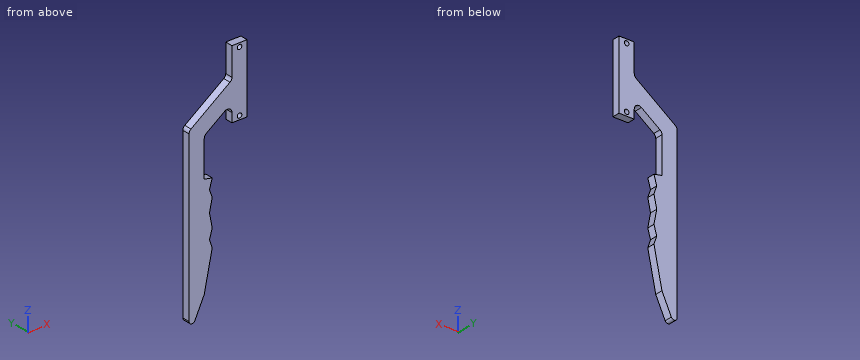
from build123d import *

# Parameters (mm, degrees)
SKETCH1_W           = 10
SKETCH1_H           = 45
BOSS_EXTRUDE1_DEPTH = 5
SKETCH2_R           = 1.5
CUT_EXTRUDE1_DEPTH  = 8
BOSS_EXTRUDE3_DEPTH = 5
BOSS_EXTRUDE4_DEPTH = 5
FILLET1_R           = 2
FILLET2_R           = 3
FILLET3_R           = 3


with BuildPart() as part:
    # Sketch1 → Boss-Extrude1 (new body)
    with BuildSketch(Plane(origin=(0, 0, 0), x_dir=(1, 0, 0), z_dir=(0, 1, 0))):
        Rectangle(SKETCH1_W, SKETCH1_H)
    extrude(amount=BOSS_EXTRUDE1_DEPTH)

    # Sketch2 → Cut-Extrude1 (cut)
    with BuildSketch(Plane(origin=(0, 5, 0), x_dir=(1, 0, 0), z_dir=(0, 1, 0))):
        with Locations(Location((0, -20, 0), (0, 0, 270))):
            Circle(SKETCH2_R)
        with Locations(Location((0, 20, 0), (0, 0, 270))):
            Circle(SKETCH2_R)
    extrude(amount=-CUT_EXTRUDE1_DEPTH, mode=Mode.SUBTRACT)

    # Sketch6 → Boss-Extrude3 (add)
    with BuildSketch(Plane(origin=(0, 5, 0), x_dir=(1, 0, 0), z_dir=(0, 1, 0))):
        Polygon((-33.227631009, 17.578800472), (-5, -2.523297008), (-5, 10.69017833), (-23.227631009, 23.670850185), (-23.227631009, 104.538936329), (-33.227631009, 104.538936329), align=None)
    extrude(amount=-BOSS_EXTRUDE3_DEPTH)

    # Sketch7 → Boss-Extrude4 (add)
    with BuildSketch(Plane(origin=(0, 5, 0), x_dir=(1, 0, 0), z_dir=(0, 1, 0))):
        Polygon((-23.227631009, 116.174137028), (-17.970128301, 90.769004099), (-19.800511719, 85.517703367), (-17.970128301, 79.310161893), (-19.800511719, 69.850883837), (-17.970128301, 61.532596279), (-19.800511719, 56.281295548), (-17.970128301, 50.073754074), (-23.227631009, 48.98573242), (-23.227631009, 104.538936329), (-33.227631009, 104.538936329), (-33.227631009, 137.531613315), align=None)
    extrude(amount=-BOSS_EXTRUDE4_DEPTH)

    # Fillet1
    fillet1_edges = [part.edges().sort_by_distance(p)[0] for p in [
        (-33.227631009, 2.5, -137.531613315),
    ]]
    fillet(fillet1_edges, radius=FILLET1_R)

    # Fillet2
    fillet2_edges = [part.edges().sort_by_distance(p)[0] for p in [
        (-5, 2.5, 2.523297008),
        (-5, 2.5, -10.69017833),
        (-23.227631009, 2.5, -23.670850185),
    ]]
    fillet(fillet2_edges, radius=FILLET2_R)

    # Fillet3
    fillet3_edges = [part.edges().sort_by_distance(p)[0] for p in [
        (-33.227631009, 2.5, -17.578800472),
    ]]
    fillet(fillet3_edges, radius=FILLET3_R)


solid = part.part
Design review of the part built by this model. Coordinates are the model's own, in mm. Round coordinates to 2 decimals unless told otherwise and drop trailing zeros. Loops run counter-clockwise (first coordinate to the right, second up) from the corner with the lowest first, then second, coordinate; pieces in that order, holes last. Notation, with made-up numbers: M 4.5,79.5 L 27.5,79.5 A21 ccw 27.5,89.5 Z; hole C 70.25,13 d9. An arc over 180 degrees is marked long. Answer as a JSON object with one key per item and string values.
Item 1: We need section D-D on z = -112. Give the boundary of the cut face in (x, y), and give its area (3 significant figures).
Answer sheet:
{"outline": "M -33.23,0 L -22.36,0 L -22.36,5 L -33.23,5 Z", "area": "54.3 mm^2"}
Item 2: We need section C-C on y = 2.45. Give the boundary of the cut face in (x, z), and give its area (3 significant figures).
Answer sheet:
{"outline": "M -33.23,-128.54 A2 ccw -29.42,-129.39 L -23.23,-116.17 L -17.97,-90.77 L -19.8,-85.52 L -17.97,-79.31 L -19.8,-69.85 L -17.97,-61.53 L -19.8,-56.28 L -17.97,-50.07 L -23.23,-48.99 L -23.23,-25.22 A3 cw -21.97,-22.77 L -9.74,-14.07 A3 cw -5,-16.51 L -5,-22.5 L 5,-22.5 L 5,22.5 L -5,22.5 L -5,4.07 A3 cw -6.26,1.63 L -31.97,-16.68 A3 ccw -33.23,-19.13 Z; hole C 0,-20 d3; hole C 0,20 d3", "area": "2,050 mm^2"}
Item 3: Wall thickness on L1, parallel to X at y = 2.55, z = 20; L2, parallel to X at y = 2.2, z = -20; L3, parallel to Z at x = -2.5, y = 0.5: over which ranges is each line inside the solid? List them lowest first. Write a range as from..to.
Answer sheet:
{"L1": "x = -5..-1.5, 1.5..5", "L2": "x = -33.23..-18.07, -5..-1.5, 1.5..5", "L3": "z = -22.5..22.5"}
Item 4: We need section B-B on z = 20. Give the boundary of the cut face in (x, y).
Answer sheet:
{"outline": "M -5,0 L -1.5,0 L -1.5,5 L -5,5 Z; M 1.5,0 L 5,0 L 5,5 L 1.5,5 Z"}
Item 5: We need section A-A on x = 0. Give the boundary of the cut face in (y, z), and give its area (3 significant figures).
Answer sheet:
{"outline": "M 0,-22.5 L 5,-22.5 L 5,-21.5 L 0,-21.5 Z; M 0,-18.5 L 5,-18.5 L 5,18.5 L 0,18.5 Z; M 0,21.5 L 5,21.5 L 5,22.5 L 0,22.5 Z", "area": "195 mm^2"}
